Design review of the part built by this model. Coordinates are the model's own, in mm. A direction names the side the tool comes from. Round coordinates to 2 decimals unless told otherwise and drop trailing zeros. Loops run counter-clockwise (first coordinate to the right, second up) from the corner with the lowest first, then second, coordinate; pieces in that order, holes last. Notation, with made-up numbers: (60.5, 77.5) - (100.5, 77.5) arc R22 cw to (100.5, 112.5) - close; hole circle Ø2 at (21.25, 31.5). An arc over 180 degrees is marked (long way). Return JSON: item names as keys, results as strings. Group by question number.
(1) We need section A-A, the plane x = -7.55. Write out the cut boundary in (y, z).
(2) Wall thickness on L1, parallel to Y at x = -7.55, z = -0.7; L2, parallel to Y at x = -19.5, z = 30; L3, parallel to X at y = 61.5, z = 3: over which ranges is each line inside the solid? List them lowest first. Write a range as [from, to].
(3) We need section D-D, the plane x = -1.5. Write out the cut boundary in (y, z), and give its area (3 significant figures).
(4) Clearance check with flat-ended pins moving along their axes: pin 1 (3 mm diameter, centred on x = -17.5, z = -0.5, fed in from -Y); pin 2 (12 mm diameter, centred on x = -6.5, y = 41, fed in from +Z); pin 3 (2 mm diameter, centred on x = -18.5, z = -1.5, fed in from +Y). State where each tip first meets the part, or that it passes through.
(5) The part is to be moulded in two halves that separate along X. For faces 1 (the cylindrical face through (-3.34, 51.35, -0.99)), 2 (the flat face through (-20, 50, 14)), 3 (the flat face through (-10, 49, -2)), say which applies: pulls with the +X half, pulls with the -X half, needs draft (parallel to the pull), parting line crosses it, or undercut.
(6) We need section B-B, the plane z = 30. Write out the cut boundary in (x, y), and give its area (3 significant figures).
(7) We need section C-C, the plane y = 27.5. Write out the cut boundary in (x, z), and give its area (3 significant figures).
(8) For faces 4 (the flat face through (-18.986, 42.527, 32.638)), 5 (the flat face through (-15.612, 5.378, -0.986)), 6 (the flat face through (-18, 78.5, -1)), list the 3-axis set-ups (+Z, -Z, +X, -X, +Y, -Y) from which the entire face can be reached by the end or side of a thin tool; tool diameter is ignored.
from build123d import *
from OCP.BRepFilletAPI import BRepFilletAPI_MakeChamfer

# Parameters (mm, degrees)
SKETCH1_W             = 100
SKETCH1_H             = 20
SKETCH1_R             = 1.6
BASE_FLANGE2_DEPTH    = 2
MITER_START           = 21.5
MITER_FLANGE1_DEPTH   = 57
MITER_FLANGE1_2_DEPTH = 1
MITER_START_2         = 77.5
MITER_FLANGE1_3_DEPTH = 1
MITER_START_3         = 22.5
MITER_FLANGE1_4_DEPTH = 55
CUT_EXTRUDE2_DEPTH    = 108.466273779
FILLET1_R             = 2.4
FILLET2_R             = 8.2
SKETCH8_R             = 2.25
CUT_EXTRUDE1_DEPTH    = 108.466273779
CHAMFER1_SIZE         = 8.9
CHAMFER1_SIZE2        = 10.606606974
CHAMFER2_SIZE         = 4


# Read off the part's stored shape, not the designer's step: Miter Flange1
# Sheet-metal steps are written as plain solids
with BuildPart() as part:
    # Sketch1 → Base-Flange2 (new body)
    with BuildSketch(Plane(origin=(0, 0, 0), x_dir=(0, 1, 0), z_dir=(0, 0, 1))):
        with Locations((50, 10)):
            Rectangle(SKETCH1_W, SKETCH1_H)
        with Locations(Location((50, 4.2, 0), (0, 0, 270))):
            Circle(SKETCH1_R, mode=Mode.SUBTRACT)
        with Locations(Location((4.2, 7.55, 0), (0, 0, 270))):
            Circle(SKETCH1_R, mode=Mode.SUBTRACT)
        with Locations(Location((95.8, 7.55, 0), (0, 0, 270))):
            Circle(SKETCH1_R, mode=Mode.SUBTRACT)
    extrude(amount=-BASE_FLANGE2_DEPTH)

    # Miter Flange1 outline → Miter Flange1 (cut)
    with BuildSketch(Plane(origin=(0, 0, 0), x_dir=(1, 0, 0), z_dir=(0, 1, 0)).offset(MITER_START)):
        with BuildLine():
            Line((-20, 0), (-19.899002398, 0))
            ThreePointArc((-19.899002398, 0), (-18.917667209, 1.443395312), (-17.2634, 2))
            Line((-17.2634, 2), (-20, 2))
            Line((-20, 2), (-20, 0))
        make_face()
    extrude(amount=MITER_FLANGE1_DEPTH, mode=Mode.SUBTRACT)

    # Miter Flange1 2 outline → Miter Flange1 2 (cut)
    with BuildSketch(Plane(origin=(0, 0, 0), x_dir=(1, 0, 0), z_dir=(0, 1, 0)).offset(MITER_START)):
        with BuildLine():
            ThreePointArc((-17.2634, 2), (-18.917667209, 1.443395312), (-19.899002398, 0))
            Line((-19.899002398, 0), (-16.2634, 0))
            Line((-16.2634, 0), (-16.2634, 2))
            Line((-16.2634, 2), (-17.2634, 2))
        make_face()
    extrude(amount=MITER_FLANGE1_2_DEPTH, mode=Mode.SUBTRACT)

    # Miter Flange1 3 outline → Miter Flange1 3 (cut)
    with BuildSketch(Plane(origin=(0, 0, 0), x_dir=(1, 0, 0), z_dir=(0, 1, 0)).offset(MITER_START_2)):
        with BuildLine():
            ThreePointArc((-17.2634, 2), (-18.917667209, 1.443395312), (-19.899002398, 0))
            Line((-19.899002398, 0), (-16.2634, 0))
            Line((-16.2634, 0), (-16.2634, 2))
            Line((-16.2634, 2), (-17.2634, 2))
        make_face()
    extrude(amount=MITER_FLANGE1_3_DEPTH, mode=Mode.SUBTRACT)

    # Miter Flange1 4 outline → Miter Flange1 4 (add)
    with BuildSketch(Plane(origin=(0, 0, 0), x_dir=(1, 0, 0), z_dir=(0, 1, 0)).offset(MITER_START_3)):
        with BuildLine():
            Line((-20, -0.7366), (-20, -35))
            Line((-20, -35), (-18, -35))
            Line((-18, -35), (-18, -0.7366))
            ThreePointArc((-18, -0.7366), (-17.784254855, -0.215745145), (-17.2634, 0))
            Line((-17.2634, 0), (-19.899002398, 0))
            ThreePointArc((-19.899002398, 0), (-19.974633029, -0.364854094), (-20, -0.7366))
        make_face()
    extrude(amount=MITER_FLANGE1_4_DEPTH)

    # Sketch9 → Cut-Extrude2 (cut, through all)
    with BuildSketch(Plane.YZ.offset(-18)):
        Polygon((22.5, 0.7366), (37.755048536, 35), (22.5, 35), align=None)
        Polygon((62.244951464, 35), (77.5, 35), (77.5, 0.7366), align=None)
        Polygon((40.4, 35), (59.6, 35), (53.657333308, 28.4), (46.342666692, 28.4), align=None)
    extrude(amount=-CUT_EXTRUDE2_DEPTH, mode=Mode.SUBTRACT)

    # Fillet1
    fillet1_edges = [part.edges().sort_by_distance(p)[0] for p in [
        (-19, 40.4, 35),
        (-19, 59.6, 35),
        (-19, 37.755048536, 35),
        (-19, 62.244951464, 35),
    ]]
    fillet(fillet1_edges, radius=FILLET1_R)

    # Fillet2
    fillet2_edges = [part.edges().sort_by_distance(p)[0] for p in [
        (-19, 53.657333308, 28.4),
        (-19, 46.342666692, 28.4),
    ]]
    fillet(fillet2_edges, radius=FILLET2_R)

    # Sketch8 → Cut-Extrude1 (cut, through all)
    with BuildSketch(Plane.YZ.offset(-18)):
        with Locations(Location((40, 30, 0), (0, 0, 270))):
            Circle(SKETCH8_R)
        with Locations(Location((60, 30, 0), (0, 0, 270))):
            Circle(SKETCH8_R)
    extrude(amount=-CUT_EXTRUDE1_DEPTH, mode=Mode.SUBTRACT)

    # Chamfer1: one chamfer whose edges measure the first distance from different faces: ONE call of the kernel's chamfer builder (chamfer() names one face for all edges)
    chamfer1_edges_1 = [part.edges().sort_by_distance(p)[0] for p in [
        (-20, 0, -1),
    ]]
    chamfer1_side_1 = [part.faces().sort_by_distance(p)[0] for p in [
        (-10, 0, -1),
    ]]
    chamfer1_edges_2 = [part.edges().sort_by_distance(p)[0] for p in [
        (-20, 100, -1),
    ]]
    chamfer1_side_2 = [part.faces().sort_by_distance(p)[0] for p in [
        (-20, 89.25, -1),
    ]]
    chamfer1 = BRepFilletAPI_MakeChamfer(part.part.solid().wrapped)
    for e in chamfer1_edges_1:
        chamfer1.Add(CHAMFER1_SIZE, CHAMFER1_SIZE2, e.wrapped, chamfer1_side_1[0].wrapped)  # the first distance lies on this face
    for e in chamfer1_edges_2:
        chamfer1.Add(CHAMFER1_SIZE, CHAMFER1_SIZE2, e.wrapped, chamfer1_side_2[0].wrapped)  # the first distance lies on this face
    add(Compound.cast(chamfer1.Shape()), mode=Mode.REPLACE)

    # Chamfer2
    chamfer2_edges = [part.edges().sort_by_distance(p)[0] for p in [
        (0, 100, -1),
        (0, 0, -1),
    ]]
    chamfer(chamfer2_edges, length=CHAMFER2_SIZE)


solid = part.part
Solutions:
{
 "1": {"outline": "(0, -2) - (2.6, -2) - (2.6, 0) - (0, 0) - close; (5.8, -2) - (94.2, -2) - (94.2, 0) - (5.8, 0) - close; (97.4, -2) - (100, -2) - (100, 0) - (97.4, 0) - close"},
 "2": {"L1": "[0, 2.6], [5.8, 94.2], [97.4, 100]", "L2": "[35.53, 37.75], [42.25, 45.13], [54.87, 57.75], [62.25, 64.47]", "L3": "[-20, -18]"},
 "3": {"outline": "(2.5, -2) - (97.5, -2) - (97.5, 0) - (2.5, 0) - close", "area": "190 mm^2"},
 "4": {"pin 1": "y = 5.84", "pin 2": "z = 0", "pin 3": "y = 93.2"},
 "5": {"face 1": "undercut", "face 2": "pulls with the -X half", "face 3": "needs draft"},
 "6": {"outline": "(-20, 35.53) - (-18, 35.53) - (-18, 37.75) - (-20, 37.75) - close; (-20, 42.25) - (-18, 42.25) - (-18, 45.13) - (-20, 45.13) - close; (-20, 54.87) - (-18, 54.87) - (-18, 57.75) - (-20, 57.75) - close; (-20, 62.25) - (-18, 62.25) - (-18, 64.47) - (-20, 64.47) - close", "area": "20.4 mm^2"},
 "7": {"outline": "(-20, 0.74) arc R2.74 ccw to (-17.26, -2) - (0, -2) - (0, 0) - (-17.26, 0) arc R0.74 cw to (-18, 0.74) - (-18, 11.97) - (-20, 11.97) - close", "area": "62.4 mm^2"},
 "8": {"face 4": "+Z, +X, -X", "face 5": "+Z, -Z, -X, -Y", "face 6": "+Z, -Z, -X"}
}
